Could you check a few things on this drawing? It's one solid part, dimensions in mm from its lowest x, y, z. Round coordinates to 2 decimals unless told otherwise and drop trailing zeros. Write each loop counter-clockwise with the first axis right and the second up, starting at its lowest first coordinate (ties: lowest second). Pieces come first, ordered by that corner, then holes. Notation, with made-up numbers: (10.25, 37) - (24.25, 37) arc R34 ccw to (24.25, 73) - close; hole circle Ø5 at (-27.5, 29). An arc over 180 degrees is marked (long way). One line per question, with ' | ' between items. Start each with the question number.
(1) Imagine slicing it at B-B (z = 13.5). Write out the boundary of the cut face in (x, y).
(2) If I drill on L1, parallel to Z at x = 2.5, y = 6; L2, parallel to Y at x = 1, z = 13.5; L3, parallel to Z at x = 4, y = 5.5 (1 decimal), over which ranges is the centre line in solid material (lowest first)?
(3) Imagine slicing it at C-C (x = 4.5). Write out the boundary of the cut face in (y, z) (1 decimal), plus the area to 3 significant figures.
(4) Imagine slicing it at D-D (y = 9). Write out the boundary of the cut face in (x, z) (3 decimals).
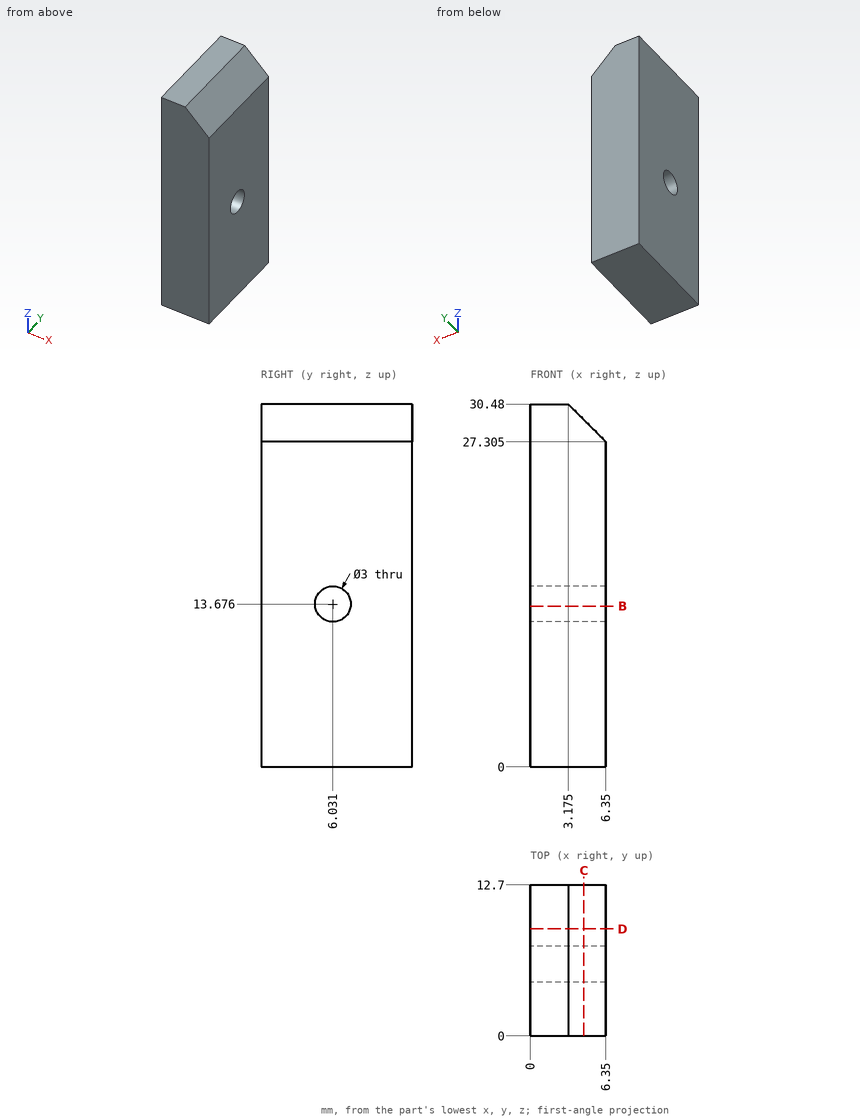
Check sheet entries:
1) outline: (0, 0) - (6.35, 0) - (6.35, 4.54) - (0, 4.54) - close; (0, 7.52) - (6.35, 7.52) - (6.35, 12.7) - (0, 12.7) - close
2) L1: 0 to 12.18, 15.18 to 30.48 | L2: 0 to 4.54, 7.52 to 12.7 | L3: 0 to 12.3, 15.1 to 29.7
3) outline: (0, 0) - (12.7, 0) - (12.7, 29.2) - (0, 29.2) - close; hole circle Ø3 at (6, 13.7) | area: 363 mm^2
4) outline: (0, 0) - (6.35, 0) - (6.35, 27.305) - (3.175, 30.48) - (0, 30.48) - close
